The drawing under review shows one solid part. Ordinate dimensions are in mm from its lowest x, y, z. A direction names the side the tool comes from. Give positions to 0.01 mm unless a question says otherwise; leave off trailing zeros. Loops run counter-clockwise (first coordinate to the right, second up) from the corner with the lowest first, then second, coordinate; pieces in that order, holes last. Notation, with made-up numbers: (38, 60) - (46, 60) arc R21 cw to (46, 65) - close; hole circle Ø10 at (10.25, 42.25). An arc over 180 degrees is marked (long way). Write each question's results on one line, items separated by ' | '.
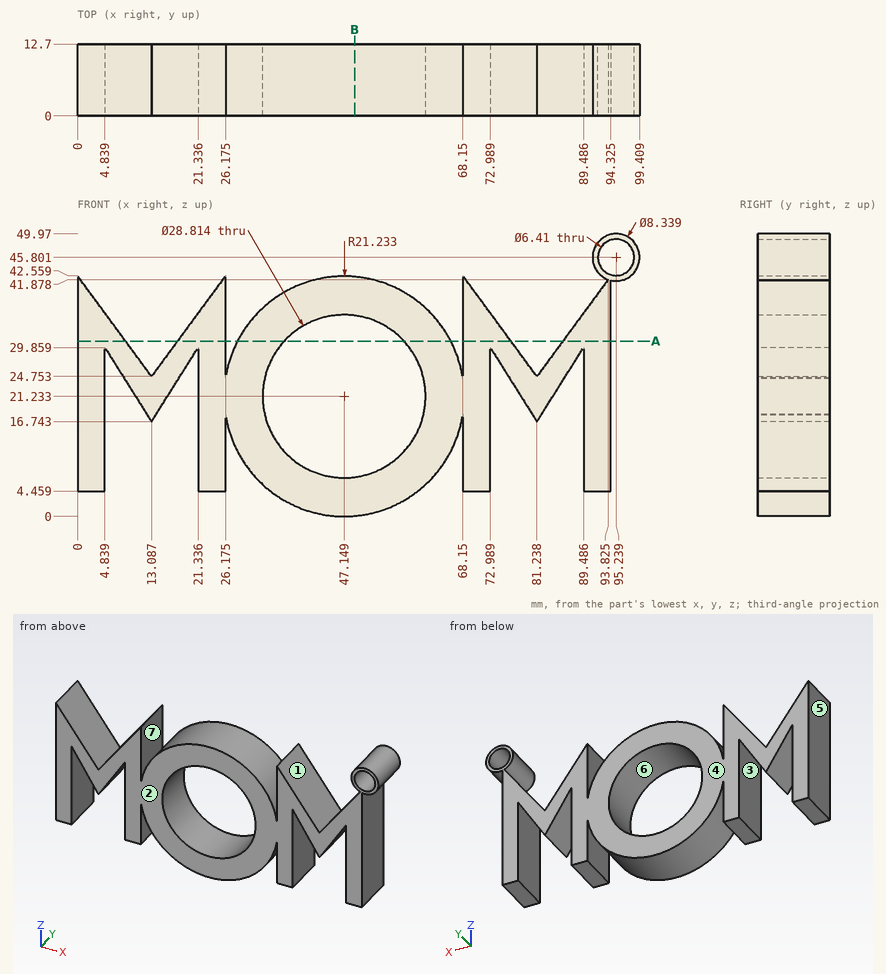
(1) Tool access review of the marked faces 1, 2 and 3: name each direction out of +Z, -Z, +X, -X, +Y, -Y from which nothing blocks a thin tool from reaching the whole face with its end or side.
Answers below:
face 1: +Z, +Y, -Y | face 2: +Z, -Z, +X, -X, -Y | face 3: -Z, +Y, -Y
(2) Draft analysis for pull direction X (two halves, no side actions). For the marked faces 4, 5, 6 and 7, state which applies: pulls with the +X half, pulls with the -X half, needs draft (parallel to the pull), parting line crosses it, or undercut.
Answers below:
face 4: needs draft | face 5: pulls with the -X half | face 6: undercut | face 7: undercut
(3) Wall thickness on line 1 along X through (y, z) = (7.25, 23.5) (1 decimal); line 2 along X through (y, z) = (3.75, 46) (1 decimal); line 3 along Z through (x, y) = (45.5, 6) (1 decimal): over which ranges is each line inside the solid? List them lowest first. Write a range as from..to.
Answers below:
line 1: 0..4.8, 8.8..17.3, 21.3..32.9, 61.4..73, 77..85.5, 89.5..94.3 | line 2: 91.1..92, 98.4..99.4 | line 3: 0.1..6.9, 35.5..42.4
(4) Take a section at B-B on x = 49. Give the boundary of the cut face in (y, z) (1 decimal), plus the area to 3 significant figures.
Answers below:
outline: (0, 0.1) - (12.7, 0.1) - (12.7, 6.9) - (0, 6.9) - close; (0, 35.5) - (12.7, 35.5) - (12.7, 42.4) - (0, 42.4) - close | area: 174 mm2
(5) Insertion check: P1, Ø5.5, axis at x = 1.5, y = 7.5, coming from the -Z side; P2, Ø4, axis at y = 7, z = 12.5, coming from the +X side (1 decimal). Each pin has a flat end and moves straight along its axis. Give the tip position at first contact, or say it passes through.
Answers below:
P1: z = 4.46 | P2: x = 94.3
(6) Take a section at A-A on z = 31. Count the separate pieces of the cut face and the enclosed holes in it.
Answers below:
separate pieces: 6 | enclosed holes: 0
